Part model, mm, in its own coordinate system. A direction names the side the tool comes from. Round coordinates to 2 decimals unless told otherwise and drop trailing zeros. Order: outer loops, then holes, each group sorted by start corner. A loop starts at its lowest first (then second) coordinate and runs counter-clockwise, first axis right, second up. Notation, with made-up numbers: (38, 15.5) - (97, 15.5) arc R17 ccw to (97, 27.5) - close; hole circle Ø10 at (48, 4). An arc over 180 degrees is marked (long way). Answer as a JSON object with one key per item and string values.
```python
from build123d import *

# Parameters (mm, degrees)
SKETCH1_R                = 21.9
BOSS_EXTRUDE3_DEPTH      = 12.5
SKETCH2_R                = 43.75
SKETCH2_R_2              = 56.25
BOSS_EXTRUDE4_DEPTH      = 18.75
BOSS_EXTRUDE4_DEPTH_BACK = 43.75
SKETCH3_R                = 14.300981298
CUT_EXTRUDE1_DEPTH       = 223.731621015


with BuildPart() as part:
    # Sketch1 → Boss-Extrude3 (new, symmetric)
    with BuildSketch(Plane(origin=(0, 0, 0), x_dir=(1, 0, 0), z_dir=(0, 1, 0))):
        with BuildLine():
            Line((-145.320623917, 56.055025997), (-150, 56.25))
            ThreePointArc((-150, 56.25), (-206.25, 0), (-150, -56.25))
            Line((-150, -56.25), (-145.320623917, -56.055025997))
            Line((-145.320623917, -56.055025997), (150, -43.75))
            ThreePointArc((150, -43.75), (193.75, 0), (150, 43.75))
            Line((150, 43.75), (-145.320623917, 56.055025997))
        make_face()
        with BuildLine():
            Line((-122.564029086, 6.3), (-114.864029086, 6.3))
            Line((-114.864029086, 6.3), (-114.864029086, -6.3))
            Line((-114.864029086, -6.3), (-122.564029086, -6.3))
            ThreePointArc((-122.564029086, -6.3), (-178.15, 0), (-122.564029086, 6.3))
        make_face(mode=Mode.SUBTRACT)
        with Locations(Location((150, 0, 0), (0, 0, 270))):
            Circle(SKETCH1_R, mode=Mode.SUBTRACT)
    extrude(amount=BOSS_EXTRUDE3_DEPTH, both=True)

    # Sketch2 → Boss-Extrude4 (add, two sides)
    with BuildSketch(Plane(origin=(0, 12.5, 0), x_dir=(1, 0, 0), z_dir=(0, 1, 0))) as boss_extrude4_sk:
        with Locations(Location((150, 0, 0), (0, 0, 270))):
            Circle(SKETCH2_R)
        with Locations(Location((-150, 0, 0), (0, 0, 270))):
            Circle(SKETCH2_R_2)
    extrude(amount=BOSS_EXTRUDE4_DEPTH)
    extrude(boss_extrude4_sk.sketch, amount=-BOSS_EXTRUDE4_DEPTH_BACK)

    # Sketch3 → Cut-Extrude1 (cut, through all)
    with BuildSketch(Plane(origin=(0, 31.25, 0), x_dir=(1, 0, 0), z_dir=(0, 1, 0))):
        with Locations(Location((150, 0, 0), (0, 0, 270))):
            Circle(SKETCH3_R)
        with BuildLine():
            Line((-114.864029086, -6.3), (-114.864029086, 6.3))
            Line((-114.864029086, 6.3), (-122.564029086, 6.3))
            ThreePointArc((-122.564029086, 6.3), (-178.15, 0), (-122.564029086, -6.3))
            Line((-122.564029086, -6.3), (-114.864029086, -6.3))
        make_face()
    extrude(amount=-CUT_EXTRUDE1_DEPTH, mode=Mode.SUBTRACT)


solid = part.part
```
Item 1: Cut at B-B (z = 0). Write the cut outline in (x, y).
Taken from the geometry:
{"outline": "(-206.25, -31.25) - (-178.15, -31.25) - (-178.15, 31.25) - (-206.25, 31.25) - close; (-114.86, -31.25) - (-93.75, -31.25) - (-93.75, -12.5) - (106.25, -12.5) - (106.25, -31.25) - (135.7, -31.25) - (135.7, 31.25) - (106.25, 31.25) - (106.25, 12.5) - (-93.75, 12.5) - (-93.75, 31.25) - (-114.86, 31.25) - close; (164.3, -31.25) - (193.75, -31.25) - (193.75, 31.25) - (164.3, 31.25) - close"}
Item 2: Probe L1, parallel to X at y = -5, z = 0; L2, parallel to X at y = -15, z = 0; L3, parallel to X at y = 19.5, z = 14.5. List the from-to ranges inside material, lowest first. Write a range as from..to.
Taken from the geometry:
{"L1": "-206.25..-178.15, -114.86..135.7, 164.3..193.75", "L2": "-206.25..-178.15, -114.86..-93.75, 106.25..135.7, 164.3..193.75", "L3": "-204.35..-174.13, -125.87..-95.65, 108.72..191.28"}
Item 3: Cut at C-C (y = 6). Write the cut outline in (x, z), plus the area to 3 significant figures.
Taken from the geometry:
{"outline": "(-145.32, -56.06) - (150, -43.75) arc R43.75 ccw to (150, 43.75) - (-145.32, 56.06) arc R56.25 ccw (long way) to start; hole (-122.56, -6.3) - (-114.86, -6.3) - (-114.86, 6.3) - (-122.56, 6.3) arc R28.15 ccw (long way) to start; hole circle Ø28.6 at (150, 0)", "area": "34,800 mm2"}
Item 4: Drop flat-ended pins along their axis: P1, Ø8, axis at x = -69.5, z = 38.5, coming from the +Y side; P2, Ø12, axis at x = -147, y = 8, coming from the -Z side; P3, Ø4, axis at x = -119, y = 9, coming from the -Z side; P4, Ø6.5, axis at y = 4, z = 1, coming from the -X side. Give the stop position or say it passes through.
Taken from the geometry:
{"P1": "y = 12.5", "P2": "z = -56.25", "P3": "z = -55.04", "P4": "x = -206.25"}
Item 5: Cut at D-D (z = -34.5). Write the cut outline in (x, y).
Taken from the geometry:
{"outline": "(-194.43, -31.25) - (-105.57, -31.25) - (-105.57, -12.5) - (123.1, -12.5) - (123.1, -31.25) - (176.9, -31.25) - (176.9, 31.25) - (123.1, 31.25) - (123.1, 12.5) - (-105.57, 12.5) - (-105.57, 31.25) - (-194.43, 31.25) - close"}
Item 6: Tool access for faces 1 (the cylindrical face through (193.378, -0.438, -5.695)), 2 (the flat face through (160.3, -31.25, -10.3)), 3 (the flat face through (-119, 0, 6.3)): list every direction of +Z, -Z, +X, -X, +Y, -Y with a clear straight run to the whole face (end or side of a thin tool).
Taken from the geometry:
{"face 1": "none", "face 2": "+Z, -Z, +X, -X, -Y", "face 3": "+Y, -Y"}
Item 7: Two-plate mould, pull along Z, no slides. Class faces 4 (the cylindrical face through (136.04, 0.44, -3.1)), 5 (the flat face through (4.407, 0.175, -49.816)), 6 (the flat face through (160.3, 31.25, -10.3)): pulls with the +Z half, pulls with the -Z half, needs draft (parallel to the pull), parting line crosses it, or undercut.
Taken from the geometry:
{"face 4": "undercut", "face 5": "pulls with the -Z half", "face 6": "needs draft"}
Item 8: Cut at A-A (y = -22.5). Write the cut outline in (x, z).
Taken from the geometry:
{"outline": "circle Ø112.5 at (-150, 0); circle Ø87.5 at (150, 0); hole (-122.56, -6.3) - (-114.86, -6.3) - (-114.86, 6.3) - (-122.56, 6.3) arc R28.15 ccw (long way) to start; hole circle Ø28.6 at (150, 0)"}
